Autodesk Inventor part; units mm, degrees
ref_plane "YZ Plane" through (0, 0, 0) normal (1, 0, 0) x (0, 1, 0)
ref_plane "XZ Plane" through (0, 0, 0) normal (0, 1, 0) x (-1, 0, 0)
ref_plane "XY Plane" through (0, 0, 0) normal (0, 0, 1) x (1, 0, 0)
sketch "Sketch2" plane through (0, 0, 0) normal (0, 0, 1) x (1, 0, 0)
  arc A0 (-24, 4) -> (-24, -4) centre (-24, 0) ccw
  arc A1 (24, -4) -> (24, 4) centre (24, 0) ccw
  line L0 (-24, 4) -> (24, 4)
  line L1 (-24, -4) -> (24, -4)
  line L2 (-39.2, 0) -> (39.2, 0)
  line L3 (0, -5.6) -> (0, 5.6)
  point P0 (0, 0)
  dimension "d0" = 4
  dimension "d1" = 4
  dimension "d2" = 48
  dimension "d3" = 0
  dimension "d4" = 24
  dimension "d9" = 180
  dimension "d10" = 0
  dimension "d98" = 48
extrude "Extrusion1" add sketch "Sketch2" along normal blind 8
sketch "Sketch11" plane through (0, 0, 8) normal (0, 0, 1) x (1, 0, 0)
  arc A0 (-24, 4) -> (-24, -4) centre (-24, 0) ccw
  circle A1 centre (-24, 0) radius 2.5
  line L0 (-39.2, 0) -> (39.2, 0)
  circle A2 centre (-16, 0) radius 2.5
  circle A3 centre (-8, 0) radius 2.5
  circle A4 centre (0, 0) radius 2.5
  circle A5 centre (8, 0) radius 2.5
  circle A6 centre (16, 0) radius 2.5
  circle A7 centre (24, 0) radius 2.5
  dimension "d99" = 5
  dimension "d105" = 8
extrude "Extrusion10" cut sketch "Sketch11" against normal through all
sketch "Sketch12" plane through (0, 0, 8) normal (0, 0, 1) x (1, 0, 0)
  circle A0 centre (24, 0) radius 2.5
  circle A1 centre (16, 0) radius 2.5
  circle A2 centre (8, 0) radius 2.5
  circle A3 centre (0, 0) radius 2.5
  circle A4 centre (-8, 0) radius 2.5
  circle A5 centre (-16, 0) radius 2.5
  circle A6 centre (-24, 0) radius 2.5
  arc A7 (-24, 4) -> (-24, -4) centre (-24, 0) ccw
  circle A8 centre (-24, 0) radius 3
  line L0 (-39.2, 0) -> (39.2, 0)
  circle A9 centre (-16, 0) radius 3
  circle A10 centre (-8, 0) radius 3
  circle A11 centre (0, 0) radius 3
  circle A12 centre (8, 0) radius 3
  circle A13 centre (16, 0) radius 3
  circle A14 centre (24, 0) radius 3
  dimension "d109" = 6
  dimension "d115" = 8
extrude "Extrusion11" cut sketch "Sketch12" against normal blind 0.8 contours L0 A14 A0 | A0 L0 A14 | A8 L0 A6 | L0 A6 A8 | A9 L0 A5 | L0 A5 A9 | A10 L0 A4 | L0 A4 A10 | A11 L0 A3 | L0 A3 A11 | A12 L0 A2 | L0 A2 A12 | A13 L0 A1 | L0 A1 A13
sketch "Sketch13" plane through (0, 0, 0) normal (0, 0, -1) x (-1, 0, 0)
  circle A0 centre (-24, 0) radius 2.5
  circle A1 centre (-16, 0) radius 2.5
  circle A2 centre (-8, 0) radius 2.5
  circle A3 centre (0, 0) radius 2.5
  circle A4 centre (8, 0) radius 2.5
  circle A5 centre (16, 0) radius 2.5
  circle A6 centre (24, 0) radius 2.5
  arc A7 (-24, 4) -> (-24, -4) centre (-24, 0) ccw
  circle A8 centre (-24, 0) radius 3
  line L0 (39.2, 0) -> (-39.2, 0)
  circle A9 centre (-16, 0) radius 3
  circle A10 centre (-8, 0) radius 3
  circle A11 centre (0, 0) radius 3
  circle A12 centre (8, 0) radius 3
  circle A13 centre (16, 0) radius 3
  circle A14 centre (24, 0) radius 3
  dimension "d119" = 6
  dimension "d125" = 8
extrude "Extrusion12" cut sketch "Sketch13" against normal blind 0.8 contours L0 A8 A0 | A0 L0 A8 | A14 L0 A6 | L0 A6 A14 | A13 L0 A5 | L0 A5 A13 | A12 L0 A4 | L0 A4 A12 | A11 L0 A3 | L0 A3 A11 | A10 L0 A2 | L0 A2 A10 | A9 L0 A1 | L0 A1 A9
sketch "Sketch14" plane through (0, 0, 8) normal (0, 0, 1) x (1, 0, 0)
  circle A0 centre (-24, 0) radius 3
  circle A1 centre (-16, 0) radius 3
  arc A2 (-24, 4) -> (-24, -4) centre (-24, 0) ccw
  line L0 (-24, 4) -> (24, 4)
  arc A3 (-22.1972, -3) -> (-22.1972, 3) centre (-24, 0) ccw
  line L1 (-22.1972, 3) -> (-17.8028, 3)
  line L2 (-22.1972, -3) -> (-17.8028, -3)
  arc A4 (-17.8028, 3) -> (-17.8028, -3) centre (-16, 0) ccw
  line L3 (-39.2, 0) -> (39.2, 0)
  arc A5 (-14.1972, -3) -> (-14.1972, 3) centre (-16, 0) ccw
  line L4 (-14.1972, 3) -> (-9.8028, 3)
  line L5 (-14.1972, -3) -> (-9.8028, -3)
  arc A6 (-9.8028, 3) -> (-9.8028, -3) centre (-8, 0) ccw
  arc A7 (-6.1972, -3) -> (-6.1972, 3) centre (-8, 0) ccw
  line L6 (-6.1972, 3) -> (-1.8028, 3)
  line L7 (-6.1972, -3) -> (-1.8028, -3)
  arc A8 (-1.8028, 3) -> (-1.8028, -3) centre (0, 0) ccw
  arc A9 (1.8028, -3) -> (1.8028, 3) centre (0, 0) ccw
  line L8 (1.8028, 3) -> (6.1972, 3)
  line L9 (1.8028, -3) -> (6.1972, -3)
  arc A10 (6.1972, 3) -> (6.1972, -3) centre (8, 0) ccw
  arc A11 (9.8028, -3) -> (9.8028, 3) centre (8, 0) ccw
  line L10 (9.8028, 3) -> (14.1972, 3)
  line L11 (9.8028, -3) -> (14.1972, -3)
  arc A12 (14.1972, 3) -> (14.1972, -3) centre (16, 0) ccw
  arc A13 (17.8028, -3) -> (17.8028, 3) centre (16, 0) ccw
  line L12 (17.8028, 3) -> (22.1972, 3)
  line L13 (17.8028, -3) -> (22.1972, -3)
  arc A14 (22.1972, 3) -> (22.1972, -3) centre (24, 0) ccw
  dimension "d129" = 7
  dimension "d131" = 7
  dimension "d137" = 8
extrude "Extrusion13" cut sketch "Sketch14" against normal through all contours A13 L12 A14 L3 | L3 A14 L13 A13 | A11 L10 A12 L3 | L3 A12 L11 A11 | A9 L8 A10 L3 | L3 A10 L9 A9 | A7 L6 A8 L3 | L3 A8 L7 A7 | A5 L4 A6 L3 | L3 A6 L5 A5 | A3 L1 A4 L3 | L3 A4 L2 A3
properties part number "7M Beam"
Input: part model. Units: mm. Frame: model coordinates. A direction names the side the tool comes from. Round coordinates to 2 decimals unless told otherwise and drop trailing zeros. Order: outer loops, then holes, each group sorted by start corner. A loop starts at its lowest first (then second) coordinate and runs counter-clockwise, first axis right, second up. Notation, with made-up numbers: (45.5, 4) - (54.5, 4) arc R15 ccw to (54.5, 9) - close; hole circle Ø2 at (12.25, -33.5). An arc over 180 degrees is marked (long way). Answer in a Markdown table with one row per item.
Item 1: Section query A-A (x = 16). Return the cut outline in (y, z), then the cut area to 3 significant figures.
Model answer:
| item | result |
|---|---|
| outline | (-4, 0) - (-3, 0) - (-3, 0.8) - (-2.5, 0.8) - (-2.5, 7.2) - (-3, 7.2) - (-3, 8) - (-4, 8) - close; (2.5, 0.8) - (3, 0.8) - (3, 0) - (4, 0) - (4, 8) - (3, 8) - (3, 7.2) - (2.5, 7.2) - close |
| area | 22.4 mm² |
Item 2: Pin query (flat end, axial travel): pin 1 (3 mm diameter, centred on x = -15, y = 0.5, fed in from -Z); pin 2 (3 mm diameter, centred on y = 3, z = 6, fed in from -X); pin 3 (1.8 mm diameter, centred on x = -17, y = -0.5, fed in from +Z); pin 4 (2 mm diameter, centred on y = -2.5, z = 7, fed in from +X). Return the tip coordinate at first contact, or that it passes through.
Model answer:
| item | result |
|---|---|
| pin 1 | stops at z = 0.8 |
| pin 2 | stops at x = -27.71 |
| pin 3 | passes through |
| pin 4 | stops at x = 27.71 |
Item 3: Mould query, pull axis Y, two halves, no side actions, for faces 4 (the cylindrical face through (28, 0, 4)), 5 (the cylindrical face through (10.385, 0.751, 4.045)), 6 (the flat face through (-2.2, 3.3, 8)). Classes: released by +Y, released by -Y, zero draft, split by the parting line, or undercut.
Model answer:
| item | result |
|---|---|
| face 4 | split by the parting line |
| face 5 | undercut |
| face 6 | zero draft |
Item 4: Reachability of faces 1 (the cylindrical face through (-26.5, 0.1, 4)), 2 (the cylindrical face through (19, 0.1, 0.4)), 3 (the cylindrical face through (10.77, -1.15, 7.61)) from +Z, -Z, +X, -X, +Y, -Y: full face, straight path, thin tool, end or side. Return the list, or none.
Model answer:
| item | result |
|---|---|
| face 1 | +Z, -Z |
| face 2 | -Z |
| face 3 | +Z |
Item 5: Section query B-B (z = 4.5). Give the number of separate pieces and of enclosed holes in the cut face, then the cut area to 3 significant figures.
Model answer:
| item | result |
|---|---|
| separate pieces | 1 |
| enclosed holes | 13 |
| area | 225 mm² |
Item 6: Line query: line 1 (Y direction, x = -3, z = 2); line 2 (Y direction, x = -8, z = 7.5); line 3 (Y direction, x = 0, z = 3.25). Output: solid intervals per line, ascending.
Model answer:
| item | result |
|---|---|
| line 1 | y = -4 to -3, -1.8 to 1.8, 3 to 4 |
| line 2 | y = -4 to -3, 3 to 4 |
| line 3 | y = -4 to -2.5, 2.5 to 4 |
